The model under review builds one solid part; all positions refer to its coordinate system, in mm. A direction names the side the tool comes from. Give positions to 0.01 mm unless a question says otherwise; leave off trailing zeros. Loops run counter-clockwise (first coordinate to the right, second up) from the corner with the lowest first, then second, coordinate; pieces in that order, holes last. Notation, with made-up numbers: M -22.5,85 L 3.5,85 A30 ccw 3.5,110 Z; hole C 40,45.5 d9. An arc over 180 degrees is marked long. One line per item, written item: value. Start each with the question number.
Q1. Mouldability with a two-part tool opening along X and no side actions: class faces 1 (the face through (-4, -103, 0)), 2 (the face through (-2, 0, -4)), 3 (the face through (-2.21, 58.53, 0.05)) as released by +X, released by -X, zero draft, split by the parting line, or undercut.
Q2. We need section B-B on y = -60. Write out the cut boundary in (x, z).
Q3. For pin 1 (1.7 mm diameter, centred on x = 3, z = 1.5, fed in from -Y); pin 2 (10 mm diameter, centred on y = -35, z = 7, fed in from -X); pin 3 (2.5 mm diameter, centred on x = 3.5, z = -2.5, fed in from -Y); pin 4 (2.5 mm diameter, centred on x = -0.5, y = -108, fed in from +Z), all flat-tipped, find the tip position at first contact; note any pin that passes through.
Q4. For faces 4 (the face through (-4, 53, 0)), 5 (the face through (-3.905, 24.65, -0.867)), 6 (the face through (4, -103, 0)), 7 (the face through (4, 53, 0)), 8 (the face through (0, -103, -3.5)), list the 3-axis set-ups (+Z, -Z, +X, -X, +Y, -Y) from which the entire face can be reached by the end or side of a thin tool; tool diameter is ignored.
Q5. To check wall thickness, follow line 1 along Y through (x, z) = (0, -0.5); line 2 along Y through (x, z) = (0.75, 0.5); line 3 along X through (y, z) = (-77, -0.25). State the ranges of each line that lie inside material, in increasing order. Write a range as from..to.
Q6. We need section A-A on x = 0. Write out the cut boundary in (y, z).
```python
from build123d import *

# Parameters (mm, degrees)
SKETCH1_R           = 4
BOSS_EXTRUDE1_DEPTH = 50
SKETCH2_R           = 9
BOSS_EXTRUDE2_DEPTH = 100
FILLET1_R           = 0.5
BOSS_EXTRUDE4_DEPTH = 3.5
BOSS_EXTRUDE6_DEPTH = 3.5
SKETCH7_R           = 3
CUT_EXTRUDE1_DEPTH  = 112.575459307
SKETCH9_R           = 3
CUT_EXTRUDE2_DEPTH  = 112.575459307


with BuildPart() as part:
    # Sketch1 → Boss-Extrude1 (new body)
    with BuildSketch(Plane(origin=(0, 0, 0), x_dir=(1, 0, 0), z_dir=(0, 1, 0))):
        with Locations(Location((0, 0, 0), (0, 0, 270))):
            Circle(SKETCH1_R)
    extrude(amount=BOSS_EXTRUDE1_DEPTH)

    # Sketch2 → Boss-Extrude2 (add)
    with BuildSketch(Plane(origin=(0, 0, 0), x_dir=(-1, 0, 0), z_dir=(0, -1, 0))):
        with Locations(Location((0, 0, 0), (0, 0, 90))):
            Circle(SKETCH2_R)
    extrude(amount=BOSS_EXTRUDE2_DEPTH)

    # Fillet1
    fillet1_edges = [part.edges().sort_by_distance(p)[0] for p in [
        (0, 0, 9),
        (0, -100, 9),
    ]]
    fillet(fillet1_edges, radius=FILLET1_R)

    # Sketch4 → Boss-Extrude4 (add, symmetric)
    with BuildSketch(Plane.XY):
        with BuildLine():
            Line((-4, -106.507163193), (-4, -100))
            Line((-4, -100), (4, -100))
            Line((4, -100), (4, -106.507163193))
            ThreePointArc((4, -106.507163193), (0, -110.507163193), (-4, -106.507163193))
        make_face()
    extrude(amount=BOSS_EXTRUDE4_DEPTH, both=True)

    # Sketch5 → Boss-Extrude6 (add, symmetric)
    with BuildSketch(Plane.XY):
        with BuildLine():
            Line((-4, 56.5), (-4, 50))
            Line((-4, 50), (4, 50))
            Line((4, 50), (4, 56.5))
            ThreePointArc((4, 56.5), (0, 60.499999816), (-4, 56.5))
        make_face()
    extrude(amount=BOSS_EXTRUDE6_DEPTH, both=True)

    # Sketch7 → Cut-Extrude1 (cut, through all)
    with BuildSketch(Plane.XY.offset(3.5)):
        with Locations((0, 56.499999816)):
            Circle(SKETCH7_R)
    extrude(amount=-CUT_EXTRUDE1_DEPTH, mode=Mode.SUBTRACT)

    # Sketch9 → Cut-Extrude2 (cut, through all)
    with BuildSketch(Plane.XY.offset(3.5)):
        with Locations((0, -106.507163193)):
            Circle(SKETCH9_R)
    extrude(amount=-CUT_EXTRUDE2_DEPTH, mode=Mode.SUBTRACT)


solid = part.part
```
Solved:
1. face 1: released by -X
1. face 2: zero draft
1. face 3: undercut
2. outline: C 0,0 d18
3. pin 1: y = -109.88
3. pin 2: x = -8.77
3. pin 3: y = -109.81
3. pin 4: through
4. face 4: +Z, -Z, -X, +Y
4. face 5: none
4. face 6: +Z, -Z, +X, -Y
4. face 7: +Z, -Z, +X, +Y
4. face 8: -Z, +X, -X, -Y
5. line 1: -110.51..-109.51, -103.51..53.5, 59.5..60.5
5. line 2: -110.44..-109.41, -103.6..53.6, 59.4..60.43
5. line 3: -9..9
6. outline: M -110.51,-3.5 L -109.51,-3.5 L -109.51,3.5 L -110.51,3.5 Z; M -103.51,-3.5 L -100,-3.5 L -100,-8.5 A0.5 ccw -99.5,-9 L -0.5,-9 A0.5 ccw 0,-8.5 L 0,-4 L 50,-4 L 50,-3.5 L 53.5,-3.5 L 53.5,3.5 L 50,3.5 L 50,4 L 0,4 L 0,8.5 A0.5 ccw -0.5,9 L -99.5,9 A0.5 ccw -100,8.5 L -100,3.5 L -103.51,3.5 Z; M 59.5,-3.5 L 60.5,-3.5 L 60.5,3.5 L 59.5,3.5 Z
